Autodesk Inventor part; units mm, degrees
ref_plane "YZ Plane" through (0, 0, 0) normal (1, 0, 0) x (0, 1, 0)
ref_plane "XZ Plane" through (0, 0, 0) normal (0, 1, 0) x (-1, 0, 0)
ref_plane "XY Plane" through (0, 0, 0) normal (0, 0, 1) x (1, 0, 0)
sketch "Sketch1" plane through (0, 0, 0) normal (0, 1, 0) x (-1, 0, 0)
  line L0 (0, -61) -> (-100, -61)
  line L1 (-100, -61) -> (-100, 0)
  line L2 (-100, 0) -> (0, 0)
  line L3 (0, 0) -> (0, -61)
  dimension "d0" = 100
  dimension "d1" = 61
extrude "Extrusion1" add sketch "Sketch1" along normal blind 2
sketch "Sketch2" plane through (0, 2, 0) normal (0, 1, 0) x (1, 0, 0)
  circle A0 centre (97.5, 57) radius 1.5
  circle A1 centre (97.5, 4) radius 1.5
  circle A2 centre (2.5, 4) radius 1.5
  circle A3 centre (2.5, 57) radius 1.5
  line L0 (100, 0) -> (100, 61)
  line L1 (100, 61) -> (0, 61)
  line L2 (0, 0) -> (100, 0)
  line L3 (0, 61) -> (0, 0)
  dimension "d4" = 2.5
  dimension "d5" = 4
  dimension "d6" = 3
  dimension "d7" = 2.5
  dimension "d8" = 4
  dimension "d9" = 4
  dimension "d10" = 2.5
  dimension "d11" = 4
  dimension "d12" = 2.5
extrude "Extrusion2" cut sketch "Sketch2" against normal blind 4 contours A0 | A1 | A2 | A3
properties part number "FSCase_Battery_Cover_v6"
Could you check a few things on this model? Use its own coordinates, in mm. Give positions to 0.01 mm unless a question says otherwise; leave off trailing zeros. Order: outer loops, then holes, each group sorted by start corner. A loop starts at its lowest first (then second) coordinate and runs counter-clockwise, first axis right, second up.
1. Suppose I cut it at B-B (z = -4). Write out the boundary of the cut face in (x, y).
Answers below:
outline: (0, 0) - (1, 0) - (1, 2) - (0, 2) - close; (4, 0) - (96, 0) - (96, 2) - (4, 2) - close; (99, 0) - (100, 0) - (100, 2) - (99, 2) - close
2. Thinking about a two-plate mould opening in X: for faces 1 (the cylindrical face through (99, 1, -4)), 2 (the flat face through (0, 1, -30)), 3 (the flat face through (100, 1, -31)), 4 (the flat face through (51, 1, 0)), which applies, +X half, -X half, draft (parallel to the pull), parting line (faces both ways), or undercut?
Answers below:
face 1: undercut
face 2: -X half
face 3: +X half
face 4: draft
3. For pin 1 (3.5 mm diameter, centred on x = 97.5, z = -57, fed in from +Y), with a flat end and sliding along its axis, tell me the tip position at first contact or that it passes through.
Answers below:
pin 1: stops at y = 2
4. Suppose I cut it at A-A (x = 2.5). Write out the boundary of the cut face in (y, z).
Answers below:
outline: (0, -61) - (2, -61) - (2, -58.5) - (0, -58.5) - close; (0, -55.5) - (2, -55.5) - (2, -5.5) - (0, -5.5) - close; (0, -2.5) - (2, -2.5) - (2, 0) - (0, 0) - close
5. I need wall thicknesses on L1, parallel to X at y = 1.1, z = -57; L2, parallel to Z at x = 2.5, y = 0.4. Which ranges of each line are inside material? Lowest first, please.
Answers below:
L1: x = 0 to 1, 4 to 96, 99 to 100
L2: z = -61 to -58.5, -55.5 to -5.5, -2.5 to 0
